Source: three-view drawing plus pictorial views. Frame: mm from the lowest corner of the part. A direction names the side the tool comes from. Coordinates: 2 decimals unless noted, no trailing zeros. Loops run counter-clockwise (first coordinate to the right, second up) from the corner with the lowest first, then second, coordinate; pieces in that order, holes last.
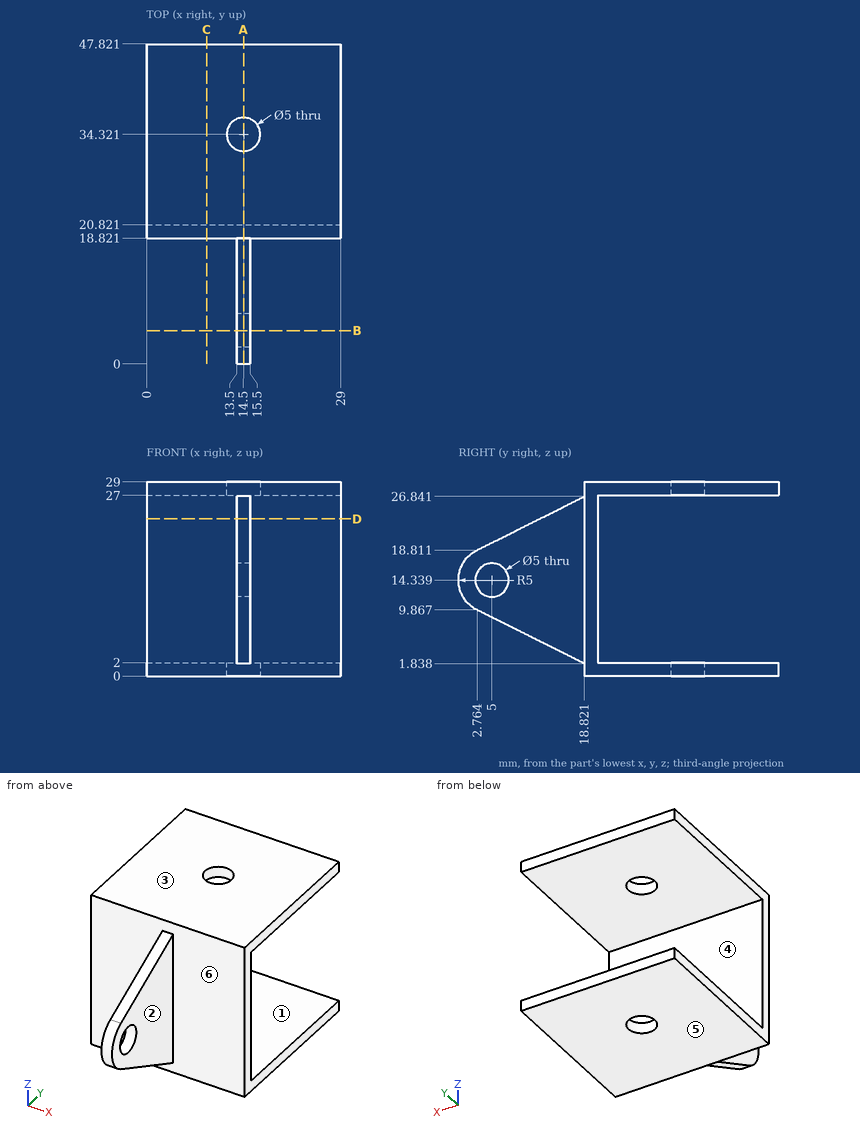
Q1. Section A-A, the plane x = 14.5. Return the cut outline in (y, z).
Q2. Section C-C, the plane x = 9. Return the cut outline in (y, z), plus the area to 3 significant figures.
Q3. Section D-D, the plane z = 23.5. Return the cut outline in (x, y).
Q4. Access query for the marked faces 1, 2 and 3. Directions: +Z, -Z, +X, -X, +Y, -Y. A direction counts if a zero-diameter tool reaches every point of the face in a straight line with its end or side. Return the directions, or none.
Q5. Draft query along Z for the marked faces 4, 5 and 6. Return one class per face: +Z half, -Z half, draft (parallel to the pull), parting line (faces both ways), or undercut.
Q6. Line query: line 1 along Z through (x, y) = (14.75, 30); line 2 along Y through (x, z) = (14.5, 27.6); line 3 along Y through (x, z) = (9, 6.75). Output: solid intervals per line, ascending.
Q7. Contact query for flat-ended pins moving along their axis: pin 1 Ø4 at (y, z) = (14.5, 25) entering from +X; pin 2 Ø5 at (x, z) = (13.5, 21) entering from -Y (1 decimal); pin 3 Ø6 at (x, z) = (12, 11) entering from -Y (1 decimal); pin 4 Ø8 at (y, z) = (31.5, 22) entering from -X. Output: stop coordinate, or through.
Q8. Section B-B, the plane y = 5. Return the cut outline in (x, z).
Derived:
1. outline: (2.76, 9.87) - (18.82, 1.84) - (18.82, 0) - (31.82, 0) - (31.82, 2) - (20.82, 2) - (20.82, 27) - (31.82, 27) - (31.82, 29) - (18.82, 29) - (18.82, 26.84) - (2.76, 18.81) arc R5 ccw to start; (36.82, 0) - (47.82, 0) - (47.82, 2) - (36.82, 2) - close; (36.82, 27) - (47.82, 27) - (47.82, 29) - (36.82, 29) - close; hole circle Ø5 at (5, 14.34)
2. outline: (18.82, 0) - (47.82, 0) - (47.82, 2) - (20.82, 2) - (20.82, 27) - (47.82, 27) - (47.82, 29) - (18.82, 29) - close
2. area: 166 mm2
3. outline: (0, 18.82) - (13.5, 18.82) - (13.5, 12.14) - (15.5, 12.14) - (15.5, 18.82) - (29, 18.82) - (29, 20.82) - (0, 20.82) - close
4. face 1: +X, -X, +Y
4. face 2: +Z, -Z, +X, -Y
4. face 3: +Z, +X, -X, +Y, -Y
5. face 4: undercut
5. face 5: -Z half
5. face 6: draft
6. line 1: z = 0 to 2, 27 to 29
6. line 2: y = 18.82 to 31.82, 36.82 to 47.82
6. line 3: y = 18.82 to 20.82
7. pin 1: stops at x = 15.5
7. pin 2: stops at y = 2.2
7. pin 3: stops at y = 0.1
7. pin 4: passes through
8. outline: (13.5, 8.75) - (15.5, 8.75) - (15.5, 11.84) - (13.5, 11.84) - close; (13.5, 16.84) - (15.5, 16.84) - (15.5, 19.93) - (13.5, 19.93) - close
